Could you check a few things on this model? Use its own coordinates, in mm. Face numbers are marked on the shaded views. A direction names the side the tool comes from. Coordinates: 2 decimals unless noted, no trailing zeros. Write each loop counter-clockwise with the first axis right and the second up, starting at its lowest first coordinate (ties: lowest second). Pieces come first, ordered by that corner, then holes.
```python
from build123d import *

# Parameters (mm, degrees)
F1_DEPTH  = 16
F2_W      = 14.5
F2_H      = 11
F3_DEPTH  = 15
F5_DEPTH  = 23.501
F7_D      = 4.2
F8_W      = 32
F8_H      = 12
F9_DEPTH  = 15
F10_R     = 5
F11_DEPTH = 25
F13_D     = 6.8


with BuildPart() as f1:
    # F0 (on Right) → F1 (new body)
    with BuildSketch(Plane.YZ):
        with BuildLine():
            ThreePointArc((0, 9.55), (9.55, 0), (0, -9.55))
            Line((0, -9.55), (-12, -9.55))
            Line((-12, -9.55), (-12, -27))
            Line((-12, -27), (20, -27))
            Line((20, -27), (20, 32))
            Line((20, 32), (-12, 32))
            Line((-12, 32), (-12, 9.55))
            Line((-12, 9.55), (0, 9.55))
        make_face()
    extrude(amount=F1_DEPTH)

    # F2 (on face) → F3 (join)
    with BuildSketch(Plane.YZ.offset(16)):
        with Locations((3.75, -21.5)):
            Rectangle(F2_W, F2_H)
    extrude(amount=F3_DEPTH)

    # F4 (on face) → F5 (cut, through all)
    with BuildSketch(Plane.XZ.offset(3.5)):
        Polygon((29.8309389108, -16), (31, -21.5), (31, -16), align=None)
    extrude(amount=-F5_DEPTH, mode=Mode.SUBTRACT)

    # F7 (through all)
    with Locations(Plane(origin=(0, 11, 0), x_dir=(-1, 0, 0), z_dir=(0, 1, 0))):
        with Locations((-26, -21.5)):
            Hole(F7_D / 2)

    # F8 (on face) → F9 (join)
    with BuildSketch(Plane.YZ.offset(16)):
        with Locations((4, 26)):
            Rectangle(F8_W, F8_H)
    extrude(amount=F9_DEPTH)

    # F10 (on face) → F11 (cut)
    with BuildSketch(Plane.XY.offset(32)):
        with Locations((8, -3)):
            Circle(F10_R)
    extrude(amount=-F11_DEPTH, mode=Mode.SUBTRACT)

    # F13 (through all)
    with Locations(Plane.YZ.offset(31)):
        with Locations((-3, 26)):
            Hole(F13_D / 2)


solid = f1.part
```
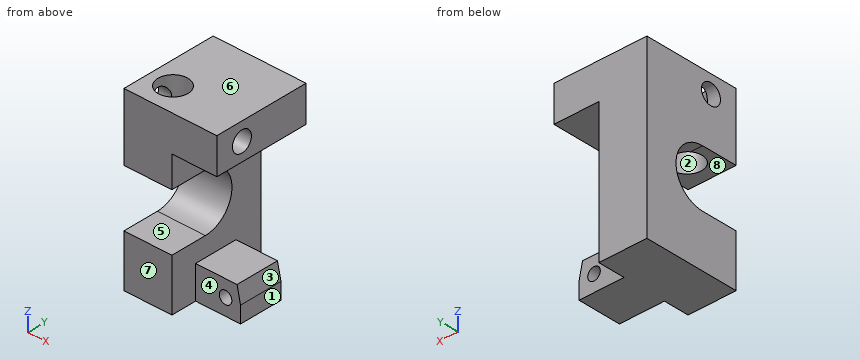
1. I want a section at B-B on z = 26. Please give me the cut outline in (x, y), plus the area to 3 significant figures.
Verdict:
outline: (0, -12) - (31, -12) - (31, -6.4) - (11.67, -6.4) arc R5 cw to (4.33, -6.4) - (0, -6.4) - close; (0, 0.4) - (4.33, 0.4) arc R5 cw to (11.67, 0.4) - (31, 0.4) - (31, 20) - (0, 20) - close
area: 765 mm2
2. I want a section at C-C on x = 8. Please give me the cut outline in (y, z), plus the area to 3 significant figures.
Verdict:
outline: (-12, -27) - (20, -27) - (20, 32) - (2, 32) - (2, 9.34) arc R9.55 cw to (0, -9.55) - (-12, -9.55) - close; (-12, 9.55) - (-8, 9.55) - (-8, 32) - (-12, 32) - close
area: 1,290 mm2
3. If we mould it in two halves opening along Z, with no side actions, what happens to the marked faces 5, 6, 7 and 8? For each: pulls with the +Z half, pulls with the -Z half, needs draft (parallel to the pull), parting line crosses it, or undercut.
Verdict:
face 5: undercut
face 6: pulls with the +Z half
face 7: needs draft
face 8: undercut
4. For pin 1 (3.5 mm diameter, centred on x = 22.5, z = -20.5, fed in from +Y); pin 2 (8 mm diameter, centred on x = 8, y = -3, fed in from +Z); pin 3 (4 mm diameter, centred on x = 25.5, y = -8, fed in from -Z); pin 4 (2 mm diameter, centred on y = 7, z = 18, fed in from -X), each with a flat end and sliding along its axis, tell me the tip position at first contact or that it passes through.
Verdict:
pin 1: stops at y = 11
pin 2: stops at z = -9.5
pin 3: stops at z = 20
pin 4: stops at x = 0
5. Please list where these lines run through material, in increasing order: line 1 along Z through (x, y) = (19.25, -3); line 2 along Z through (x, y) = (2.8, -3); line 3 along Y through (x, z) = (3.1, 26).
Verdict:
line 1: z = -27 to -16, 20 to 22.6, 29.4 to 32
line 2: z = -27 to -9.55, 9.55 to 22.6, 29.4 to 32
line 3: y = -12 to -6.4, 0.4 to 20
6. I want a section at A-A on x = 26. Please give me the cut outline in (y, z).
Verdict:
outline: (-12, 20) - (20, 20) - (20, 32) - (-12, 32) - close; (-3.5, -27) - (11, -27) - (11, -23.6) - (-3.5, -23.6) - close; (-3.5, -19.4) - (11, -19.4) - (11, -16) - (-3.5, -16) - close; hole circle Ø6.8 at (-3, 26)
7. I want a section at D-D on y = 5.5. Please give me the cut outline in (x, z), plus the area to 3 significant figures.
Verdict:
outline: (0, -27) - (31, -27) - (31, -21.5) - (29.83, -16) - (16, -16) - (16, -7.81) - (0, -7.81) - close; (0, 7.81) - (16, 7.81) - (16, 20) - (31, 20) - (31, 32) - (0, 32) - close; hole circle Ø4.2 at (26, -21.5)
area: 1,020 mm2
8. On a 3-axis mill with a long thin cutter (end or side, diameter ignored), from which of +Z, -Z, +X, -X, +Y, -Y can I reach the whole of each face in a straight line? I mean the marked faces 1, 2, 3 and 4. Say none if no direction works.
Verdict:
face 1: +Z, -Z, +X, +Y, -Y
face 2: +Z
face 3: +X, +Y, -Y
face 4: -Z, +X, -Y
